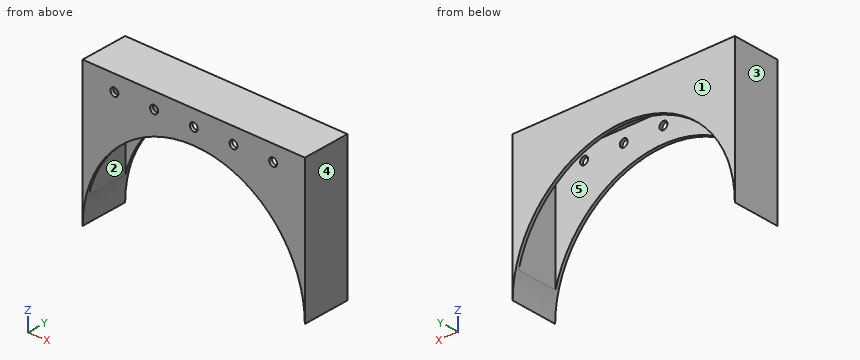
```python
from build123d import *

# Parameters (mm, degrees)
F0_R     = 2.5
F1_DEPTH = 30
F2_T     = -2
F3_DEPTH = 5


with BuildPart() as f1:
    # F0 (on Front) → F1 (new body)
    with BuildSketch(Plane.XZ):
        with BuildLine():
            ThreePointArc((-70, 0), (0, 70), (70, 0))
            Line((70, 0), (70, 90))
            Line((70, 90), (-70, 90))
            Line((-70, 90), (-70, 0.4057721722))
            Line((-70, 0.4057721722), (-70, 0))
        make_face()
        with Locations((-50, 80)):
            Circle(F0_R, mode=Mode.SUBTRACT)
        with Locations((-25, 80)):
            Circle(F0_R, mode=Mode.SUBTRACT)
        with Locations((0, 80)):
            Circle(F0_R, mode=Mode.SUBTRACT)
        with Locations((25, 80)):
            Circle(F0_R, mode=Mode.SUBTRACT)
        with Locations((50, 80)):
            Circle(F0_R, mode=Mode.SUBTRACT)
        with Locations((50, 80)):
            Circle(F0_R)
        with Locations((25, 80)):
            Circle(F0_R)
        with Locations((0, 80)):
            Circle(F0_R)
        with Locations((-25, 80)):
            Circle(F0_R)
        with Locations((-50, 80)):
            Circle(F0_R)
    extrude(amount=-F1_DEPTH)

    # F2
    f2_openings = [f1.faces().sort_by_distance(p)[0] for p in [
        (0, 15, 70),
    ]]
    offset(amount=F2_T, openings=f2_openings, kind=Kind.INTERSECTION)

    # F0 (on Front) → F3 (cut)
    with BuildSketch(Plane.XZ):
        with Locations((50, 80)):
            Circle(F0_R)
        with Locations((25, 80)):
            Circle(F0_R)
        with Locations((0, 80)):
            Circle(F0_R)
        with Locations((-25, 80)):
            Circle(F0_R)
        with Locations((-50, 80)):
            Circle(F0_R)
    extrude(amount=-F3_DEPTH, mode=Mode.SUBTRACT)


solid = f1.part
```
The model under review builds one solid part; all positions refer to its coordinate system, in mm. Face numbers are marked on the shaded views. A direction names the side the tool comes from. Round coordinates to 2 decimals unless told otherwise and drop trailing zeros. Write each loop counter-clockwise with the first axis right and the second up, starting at its lowest first coordinate (ties: lowest second). Pieces come first, ordered by that corner, then holes.
(1) We need section A-A on x = 0. Give the boundary of the cut face in (y, z), and give its area (3 significant figures).
(2) Machinability: for the marked faces 4 and 5, which of the approach directions +Z, -Z, +X, -X, +Y, -Y give a long, thin tool a straight path to every point of the face, cutting with its end or side? Answer none if there is none.
(3) Insertion check: pin 1 (13 mm diameter, centred on x = -22.5, y = 9.5, fed in from -Z); pin 2 (4 mm diameter, centred on x = 25, z = 80, fed in from -Y); pin 3 (10 mm diameter, centred on x = 22, y = 6, fed in from -Z). Each pin has a flat end and moves straight along its axis. Give the tip position at first contact, or say it passes through.
(4) We need section D-D on x = 30. Give the boundary of the cut face in (y, z), and give its area (3 significant figures).
(5) Wall thickness on L1, parallel to X at y = 18.5, z = 52; L2, parallel to Y at x = -51.5, z = 66; L3, parallel to Z at x = -25, y = 0.5: over which ranges is each line inside the solid? List them lowest first.
(6) We need section B-B on z = 59. Give the boundary of the cut face in (x, y), and give its area (3 significant figures).
(7) We need section C-C on y = 9. Give the boundary of the cut face in (x, z), and give its area (3 significant figures).
(8) Mouldability with a two-part tool opening along X and no side actions: class the marked faces 1, 2 and 3 as +X half, -X half, draft (parallel to the pull), parting line (faces both ways), or undercut.
Findings below:
1. outline: (0, 70) - (2, 70) - (2, 77.5) - (0, 77.5) - close; (0, 82.5) - (2, 82.5) - (2, 88) - (28, 88) - (28, 70) - (30, 70) - (30, 90) - (0, 90) - close
1. area: 122 mm2
2. face 4: +Z, -Z, +X, +Y, -Y
2. face 5: -Z
3. pin 1: stops at z = 88
3. pin 2: stops at y = 28
3. pin 3: stops at z = 65.38
4. outline: (0, 63.25) - (2, 63.25) - (2, 88) - (28, 88) - (28, 63.25) - (30, 63.25) - (30, 90) - (0, 90) - close
4. area: 159 mm2
5. L1: x = -70 to -68, 68 to 70
5. L2: y = 0 to 2, 28 to 30
5. L3: z = 65.38 to 77.5, 82.5 to 90
6. outline: (-70, 0) - (-37.67, 0) - (-37.67, 2) - (-68, 2) - (-68, 28) - (-37.67, 28) - (-37.67, 30) - (-70, 30) - close; (37.67, 0) - (70, 0) - (70, 30) - (37.67, 30) - (37.67, 28) - (68, 28) - (68, 2) - (37.67, 2) - close
6. area: 363 mm2
7. outline: (-70, 0) arc R70 cw to (-68, 16.61) - (-68, 88) - (68, 88) - (68, 16.61) arc R70 cw to (70, 0) - (70, 90) - (-70, 90) - close
7. area: 588 mm2
8. face 1: draft
8. face 2: undercut
8. face 3: -X half
